```python
from build123d import *

# Parameters (mm, degrees)
SKETCH_W  = 95
SKETCH_H  = 70
SKETCH_R  = 9.5
PAD_DEPTH = 10


with BuildPart() as part:
    # Sketch → Pad (new body)
    with BuildSketch(Plane.XY):
        with Locations((27.5, -15)):
            Rectangle(SKETCH_W, SKETCH_H)
        with Locations((0, -30)):
            Circle(SKETCH_R, mode=Mode.SUBTRACT)
        with BuildLine():
            ThreePointArc((-5, -6.244998), (8, 0), (-5, 6.244998))
            Line((-5, 9), (-5, 6.244998))
            Line((-8.125, 9), (-5, 9))
            Line((-8.125, -9), (-8.125, 9))
            Line((-5, -9), (-8.125, -9))
            Line((-5, -6.244998), (-5, -9))
        make_face(mode=Mode.SUBTRACT)
    extrude(amount=PAD_DEPTH)


solid = part.part
```
Read the model definition and answer for the solid it produces. Units are mm, in the model's axes. A direction names the side the tool comes from. Round coordinates to 2 decimals unless told otherwise and drop trailing zeros. Write each loop counter-clockwise with the first axis right and the second up, starting at its lowest first coordinate (ties: lowest second). Pieces come first, ordered by that corner, then holes. Notation, with made-up numbers: (78.25, -2.5) - (111.25, -2.5) arc R14 cw to (111.25, 22.5) - close; hole circle Ø2 at (-15, -0.75). An arc over 180 degrees is marked (long way). Use CSV: the item, a comma, the result in double quotes.
Q1. Find section C-C, the plane z = 8.25. Write down the section's boundary in (x, y) (3 decimals).
Values:
outline,"(-20, -50) - (75, -50) - (75, 20) - (-20, 20) - close; hole circle Ø19 at (0, -30); hole (-8.125, -9) - (-5, -9) - (-5, -6.245) arc R8 ccw (long way) to (-5, 6.245) - (-5, 9) - (-8.125, 9) - close"
Q2. Find section B-B, the plane y = -30. Write down the section's boundary in (x, z).
Values:
outline,"(-20, 0) - (-9.5, 0) - (-9.5, 10) - (-20, 10) - close; (9.5, 0) - (75, 0) - (75, 10) - (9.5, 10) - close"
Q3. Find section D-D, the plane y = 0. Write down the section's boundary in (x, z) (3 decimals).
Values:
outline,"(-20, 0) - (-8.125, 0) - (-8.125, 10) - (-20, 10) - close; (8, 0) - (75, 0) - (75, 10) - (8, 10) - close"
Q4. Straight lines are drawn through the part: line 1 along Y through (x, z) = (0, 7.5); line 2 along X through (y, z) = (0, 4.75) (3 decimals); line 3 along X through (y, z) = (-5, 7.25) (3 decimals). For each, find the intervals that lie inside material, in ascending order.
Values:
line 1,"y = -50 to -39.5, -20.5 to -8, 8 to 20"
line 2,"x = -20 to -8.125, 8 to 75"
line 3,"x = -20 to -8.125, 6.245 to 75"
Q5. A tool of negligible diameter and unlimited length cuts with its end or side. For faces 1 (the flat face through (-5, 8, 5)), 2 (the flat face through (27, 20, 5)), from which of +Z, -Z, +X, -X, +Y, -Y can it reach the whole face along a straight path? Write none if from no direction.
Values:
face 1,"+Z, -Z"
face 2,"+Z, -Z, +X, -X, +Y"
Q6. Find section A-A, the plane x = 0. Write down the section's boundary in (y, z).
Values:
outline,"(-50, 0) - (-39.5, 0) - (-39.5, 10) - (-50, 10) - close; (-20.5, 0) - (-8, 0) - (-8, 10) - (-20.5, 10) - close; (8, 0) - (20, 0) - (20, 10) - (8, 10) - close"
Q7. Determine the mould class of faces 3 (the flat face through (-20, -15, 5)), 4 (the flat face through (27, -50, 5)), 5 (the flat face through (-7, -9, 5)) for opening direction Y: +Y half, -Y half, draft (parallel to the pull), parting line (faces both ways), or undercut.
Values:
face 3,"draft"
face 4,"-Y half"
face 5,"undercut"
